Work out the finished part from the listing and answer in its coordinate system (mm). Face numbers are marked on the shaded views. A direction names the side the tool comes from. Round coordinates to 2 decimals unless told otherwise and drop trailing zeros. Write each loop counter-clockwise with the first axis right and the second up, starting at its lowest first coordinate (ties: lowest second). Pieces come first, ordered by that corner, then holes.
1. Find section B-B (x = 47). Write down the section's boundary in (y, z).
2. Straight lines are drawn through the part: probe 1 along Y at (x, z) = (159.5, -15); probe 2 along X at (y, z) = (-189, -16.5); probe 3 along X at (y, z) = (130, -7.25). For each, find the intervals that lie inside material, in ascending order.
3. Determine the mould class of the marked faces 1 and 2 for opening direction X: pulls with the +X half, pulls with the -X half, needs draft (parallel to the pull), parting line crosses it, or undercut.
4. Flat-ended cylindrical pins translate along their axes: pin 1 Ø4 at (y, z) = (-45, -8.5) entering from +X; pin 2 Ø6 at (x, z) = (107, -14.5) entering from -Y; pin 3 Ø8 at (y, z) = (148, 6) entering from -X. Find the tip coordinate at first contact, or state that the pin passes through.
5. Find section A-A (y = 47.5). Write down the section's boundary in (x, z).
6. A tool of negligible diameter and unlimited length cuts with its end or side. For the marked faces 3, 4, 5, 6 and 7, from which of +Z, -Z, +X, -X, +Y, -Y can it reach the whole face along a straight path? Write none if from no direction.
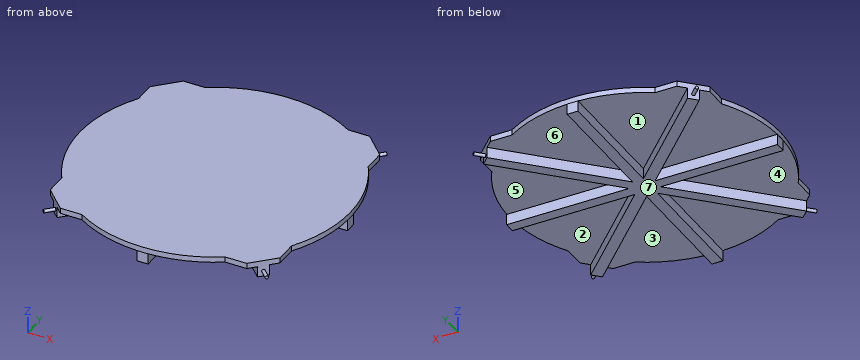
```python
from build123d import *

# Parameters (mm, degrees)
BOSS_EXTRUDE2_DEPTH = 10
BOSS_EXTRUDE3_DEPTH = 20
SKETCH3_R           = 3
BOSS_EXTRUDE4_DEPTH = 20
SKETCH4_R           = 3
BOSS_EXTRUDE5_DEPTH = 20
SKETCH5_R           = 3
BOSS_EXTRUDE6_DEPTH = 20
BOSS_EXTRUDE7_START = 20
SKETCH8_R           = 3
BOSS_EXTRUDE7_DEPTH = 20


with BuildPart() as part:
    # Sketch1 → Boss-Extrude2 (new body)
    with BuildSketch(Plane.XY):
        with BuildLine():
            Line((-172.132034356, 212.132034356), (-132.287565553, 212.132034356))
            ThreePointArc((-132.287565553, 212.132034356), (0, 250), (132.287565553, 212.132034356))
            Line((132.287565553, 212.132034356), (172.132034356, 212.132034356))
            Line((172.132034356, 212.132034356), (212.132034356, 172.132034356))
            Line((212.132034356, 172.132034356), (212.132034356, 132.287565553))
            ThreePointArc((212.132034356, 132.287565553), (250, 0), (212.132034356, -132.287565553))
            Line((212.132034356, -132.287565553), (212.132034356, -172.132034356))
            Line((212.132034356, -172.132034356), (172.132034356, -212.132034356))
            Line((172.132034356, -212.132034356), (132.287565553, -212.132034356))
            ThreePointArc((132.287565553, -212.132034356), (0, -250), (-132.287565553, -212.132034356))
            Line((-132.287565553, -212.132034356), (-172.132034356, -212.132034356))
            Line((-172.132034356, -212.132034356), (-212.132034356, -172.132034356))
            Line((-212.132034356, -172.132034356), (-212.132034356, -132.287565553))
            ThreePointArc((-212.132034356, -132.287565553), (-250, 0), (-212.132034356, 132.287565553))
            Line((-212.132034356, 132.287565553), (-212.132034356, 172.132034356))
            Line((-212.132034356, 172.132034356), (-172.132034356, 212.132034356))
        make_face()
    extrude(amount=BOSS_EXTRUDE2_DEPTH)

    # Sketch2 → Boss-Extrude3 (add)
    with BuildSketch(Plane(origin=(0, 0, 0), x_dir=(-1, 0, 0), z_dir=(0, 0, -1))):
        Polygon((10, 250), (-10, 250), (-10, 24.142135624), (-185.060966544, 199.203102168), (-199.203102168, 185.060966544), (-24.142135624, 10), (-250, 10), (-250, -10), (-24.142135624, -10), (-199.203102168, -185.060966544), (-185.060966544, -199.203102168), (-10, -24.142135624), (-10, -249.799919936), (10, -249.799919936), (10, -24.142135624), (185.060966544, -199.203102168), (199.203102168, -185.060966544), (24.142135624, -10), (249.799919936, -10), (249.799919936, 10), (24.142135624, 10), (199.203102168, 185.060966544), (192.132034356, 192.132034356), (185.060966544, 199.203102168), (10, 24.142135624), align=None)
    extrude(amount=BOSS_EXTRUDE3_DEPTH)

    # Sketch3 → Boss-Extrude4 (add)
    with BuildSketch(Plane(origin=(192.132034356, 192.132034356, 0), x_dir=(0, 0, -1), z_dir=(0.7071067811865465, 0.7071067811865487, 0))):
        with Locations(Location((9.977178016, 0, 0), (0, 0, 90))):
            Circle(SKETCH3_R)
    extrude(amount=BOSS_EXTRUDE4_DEPTH)

    # Sketch4 → Boss-Extrude5 (add)
    with BuildSketch(Plane(origin=(-192.132034356, 192.132034356, 0), x_dir=(0, 0, 1), z_dir=(-0.707106781186549, 0.707106781186546, 0))):
        with Locations(Location((-10, 0, 0), (0, 0, 270))):
            Circle(SKETCH4_R)
    extrude(amount=BOSS_EXTRUDE5_DEPTH)

    # Sketch5 → Boss-Extrude6 (add)
    with BuildSketch(Plane(origin=(-192.132034356, -192.132034356, 0), x_dir=(0, 0, 1), z_dir=(-0.7071067811865456, -0.7071067811865495, 0))):
        with Locations(Location((-10, 0, 0), (0, 0, 90))):
            Circle(SKETCH5_R)
    extrude(amount=BOSS_EXTRUDE6_DEPTH)

    # Sketch8 → Boss-Extrude7 (add)
    with BuildSketch(Plane(origin=(192.132034356, -192.132034356, 0), x_dir=(0, 0, -1), z_dir=(0.7071067811865489, -0.7071067811865462, 0)).offset(BOSS_EXTRUDE7_START)):
        with Locations(Location((10, 0, 0), (0, 0, 270))):
            Circle(SKETCH8_R)
    extrude(amount=-BOSS_EXTRUDE7_DEPTH)


solid = part.part
```
Worked answers:
1. outline: (-245.54, 0) - (-61.14, 0) - (-61.14, -20) - (-32.86, -20) - (-32.86, 0) - (-10, 0) - (-10, -20) - (10, -20) - (10, 0) - (32.86, 0) - (32.86, -20) - (61.14, -20) - (61.14, 0) - (245.54, 0) - (245.54, 10) - (-245.54, 10) - close
2. probe 1: y = -173.64 to -145.36, -10 to 10, 145.36 to 173.64
2. probe 2: x = -195.26 to -174.86, -10 to 10, 174.86 to 195.26
2. probe 3: x = -144.14 to -115.86, -10 to 10, 115.86 to 144.14
3. face 1: undercut
3. face 2: needs draft
4. pin 1: stops at x = 61.14
4. pin 2: stops at y = -124.14
4. pin 3: stops at x = -212.13
5. outline: (-245.45, 0) - (-61.64, 0) - (-61.64, -20) - (-33.36, -20) - (-33.36, 0) - (-10, 0) - (-10, -20) - (10, -20) - (10, 0) - (33.36, 0) - (33.36, -20) - (61.64, -20) - (61.64, 0) - (245.45, 0) - (245.45, 10) - (-245.45, 10) - close
6. face 3: -Z, -Y
6. face 4: -Z, -X
6. face 5: -Z, +X
6. face 6: -Z, +Y
6. face 7: -Z, +X, -X, +Y, -Y
